Input: part model. Units: mm. Frame: model coordinates. Face numbers are marked on the shaded views. A direction names the side the tool comes from. Coordinates: 2 decimals unless noted, no trailing zeros. Loops run counter-clockwise (first coordinate to the right, second up) from the corner with the lowest first, then second, coordinate; pieces in that order, holes last. Notation, with made-up numbers: (63, 72.5) - (119, 72.5) arc R6 cw to (119, 77.5) - close; hole circle Ø1 at (53, 68.5). An arc over 180 degrees is marked (long way). Write item = value, one per line. Start each with the question number.
from build123d import *

# Parameters (mm, degrees)
BOSS_EXTRUDE1_DEPTH     = 9.525
CUT_EXTRUDE4_DEPTH      = 143.309436177
CUT_EXTRUDE4_DEPTH_BACK = 143.309436177
SKETCH3_W               = 7.62
SKETCH3_H               = 30.142095215
CUT_EXTRUDE6_DEPTH      = 142.563704741
CUT_EXTRUDE6_DEPTH_BACK = 142.563704741
SKETCH5_R               = 6.35


with BuildPart() as part:
    # Sketch1 → Boss-Extrude1 (new, symmetric)
    with BuildSketch(Plane.YZ):
        with BuildLine():
            Line((0, 12.7), (127, 12.7))
            ThreePointArc((127, 12.7), (139.7, 0), (127, -12.7))
            Line((127, -12.7), (0, -12.7))
            ThreePointArc((0, -12.7), (-12.7, 0), (0, 12.7))
        make_face()
    extrude(amount=BOSS_EXTRUDE1_DEPTH, both=True)

    # Sketch3 → Cut-Extrude4 (cut, two sides: drawn at the far end of the back side and taken through both)
    with BuildSketch(Plane.XY.offset(12.7).offset(-CUT_EXTRUDE4_DEPTH_BACK)):
        with Locations((0, 132.016308081)):
            Rectangle(SKETCH3_W, SKETCH3_H)
        with Locations((0, -5.601173979)):
            Rectangle(SKETCH3_W, SKETCH3_H)
    extrude(amount=CUT_EXTRUDE4_DEPTH + CUT_EXTRUDE4_DEPTH_BACK, mode=Mode.SUBTRACT)

    # Sketch5 → Cut-Extrude6 (cut, two sides: drawn at the far end of the back side and taken through both)
    with BuildSketch(Plane.YZ.offset(9.525).offset(-CUT_EXTRUDE6_DEPTH_BACK)):
        with Locations(Location((0, 0, 0), (0, 0, 270))):
            Circle(SKETCH5_R)
        with Locations(Location((127, 0, 0), (0, 0, 270))):
            Circle(SKETCH5_R)
    extrude(amount=CUT_EXTRUDE6_DEPTH + CUT_EXTRUDE6_DEPTH_BACK, mode=Mode.SUBTRACT)


solid = part.part
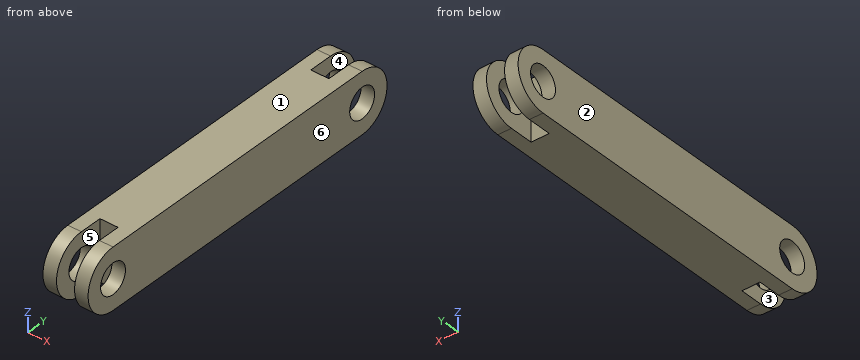
Item 1: Cut plane C-C on z = 10.5. Return loops of the section in (x, y) (3 decimals).
Item 2: Ray query, line 1 (Y direction, x = -6.8, z = 0); line 2 (Z direction, x = 7.45, y = 127); line 3 (X direction, y = 9, z = -5) (3 decimals). Return the intervals inside material, ascending.
Item 3: Cut plane B-B on x = -6.25. Return loops of the section in (y, z), plus the area to 3 significant figures.
Item 4: Pull-direction query (X, two-part tool) for the marked faces 1, 2 and 3; classes: pulls with the +X half, pulls with the -X half, needs draft (parallel to the pull), parting line crosses it, or undercut.
Item 5: Pin query (flat end, axial travel): pin 1 (2.5 mm diameter, centred on x = 0, z = 2, fed in from -Y); pin 2 (8 mm diameter, centred on x = 2.5, z = 5, fed in from +Y); pin 3 (1 mm diameter, centred on x = 1.5, z = -8, fed in from +Y). Return the tip coordinate at first contact, or that it passes through.
Item 6: Cut plane D-D on x = 0.5. Return loops of the section in (y, z), plus the area to 3 significant figures.
Item 7: Access query for the marked faces 4, 5 and 6. Directions: +Z, -Z, +X, -X, +Y, -Y. A direction counts if a zero-diameter tool reaches every point of the face in a straight line with its end or side. Return the directions, or none.
Item 8: Cut plane A-A on z = 0. Return loops of the section in (x, y) (3 decimals).
Recorded:
q1.outline = (-9.525, -7.144) - (-3.81, -7.144) - (-3.81, 9.47) - (3.81, 9.47) - (3.81, -7.144) - (9.525, -7.144) - (9.525, 134.144) - (3.81, 134.144) - (3.81, 116.945) - (-3.81, 116.945) - (-3.81, 134.144) - (-9.525, 134.144) - close
q2.line_1 = -12.7 to -6.35, 6.35 to 120.65, 133.35 to 139.7
q2.line_2 = -12.7 to -6.35, 6.35 to 12.7
q2.line_3 = -9.525 to -3.81, 3.81 to 9.525
q3.outline = (0, -12.7) - (127, -12.7) arc R12.7 ccw to (127, 12.7) - (0, 12.7) arc R12.7 ccw to start; hole circle Ø12.7 at (0, 0); hole circle Ø12.7 at (127, 0)
q3.area = 3,480 mm²
q4.face_1 = needs draft
q4.face_2 = pulls with the -X half
q4.face_3 = undercut
q5.pin_1 = 9.47
q5.pin_2 = 139.64
q5.pin_3 = 116.95
q6.outline = (9.47, -12.7) - (116.95, -12.7) - (116.95, 12.7) - (9.47, 12.7) - close
q6.area = 2,730 mm²
q7.face_4 = +Z, -Z, +Y
q7.face_5 = +Z, -Z, -Y
q7.face_6 = +Z, -Z, +X, +Y, -Y
q8.outline = (-9.525, -12.7) - (-3.81, -12.7) - (-3.81, -6.35) - (-9.525, -6.35) - close; (-9.525, 6.35) - (-3.81, 6.35) - (-3.81, 9.47) - (3.81, 9.47) - (3.81, 6.35) - (9.525, 6.35) - (9.525, 120.65) - (3.81, 120.65) - (3.81, 116.945) - (-3.81, 116.945) - (-3.81, 120.65) - (-9.525, 120.65) - close; (-9.525, 133.35) - (-3.81, 133.35) - (-3.81, 139.7) - (-9.525, 139.7) - close; (3.81, -12.7) - (9.525, -12.7) - (9.525, -6.35) - (3.81, -6.35) - close; (3.81, 133.35) - (9.525, 133.35) - (9.525, 139.7) - (3.81, 139.7) - close
